Here's how the part is built. I have some questions about the finished solid (model axes, mm). Round coordinates to 2 decimals unless told otherwise and drop trailing zeros. Loops run counter-clockwise (first coordinate to the right, second up) from the corner with the lowest first, then second, coordinate; pieces in that order, holes last. Notation, with made-up numbers: M 74.25,6.5 L 120.25,6.5 A20 cw 120.25,38.5 Z; hole C 47,-23.5 d3. An arc over 180 degrees is marked long. Write item = value, one per line. Start each with the question number.
from build123d import *

# Parameters (mm, degrees)
F0_W     = 50
F0_H     = 80
F1_DEPTH = 10
F2_R     = 9
F3_DEPTH = 10.001
F4_R     = 5


with BuildPart() as f1:
    # F0 (on Front) → F1 (new body)
    with BuildSketch(Plane.XZ):
        with Locations((25, -40)):
            Rectangle(F0_W, F0_H)
    extrude(amount=F1_DEPTH)

    # F2 (on face) → F3 (cut, through all)
    with BuildSketch(Plane.XZ.offset(10)):
        with Locations((25, -40)):
            Circle(F2_R)
    extrude(amount=-F3_DEPTH, mode=Mode.SUBTRACT)

    # F4
    f4_edges = [f1.edges().sort_by_distance(p)[0] for p in [
        (50, -5, 0),
        (0, -5, 0),
        (50, -5, -80),
        (0, -5, -80),
    ]]
    fillet(f4_edges, radius=F4_R)


solid = f1.part
Item 1: Please list where these lines run through material, in increasing order: line 1 (Z direction, x = 25, y = -6.5); line 2 (Z direction, x = 32, y = -7.25); line 3 (X direction, y = -3.75, z = -41.5). Write a range as [from, to].
Item 2: I want a section at B-B, the plane y = -5.75. List the corners of the cut face in (x, z) for me.
Item 3: I want a section at A-A, the plane z = -40. List the corners of the cut face in (x, y) for me, then the cut area to 3 significant figures.
Item 4: We'd pull the mould along X, two halves only. Please class faces 1 (the cylindrical face through (29.84, -5.07, -32.41)), 2 (the flat face through (25, -5, 0)), 3 (the flat face through (50, -5, -40)): released by +X, released by -X, zero draft, split by the parting line, or undercut.
Item 5: I want a section at C-C, the plane x = 25. List the corners of the cut face in (y, z) for me.
Item 6: Will this pin go through, and if not, where does the flat tip stop? pin 1 Ø23.5 at (x, z) = (25, -40) entering from +Y.
Worked out:
q1.line_1 = [-80, -49], [-31, 0]
q1.line_2 = [-80, -45.66], [-34.34, 0]
q1.line_3 = [0, 16.13], [33.87, 50]
q2.outline = M 0,-75 A5 ccw 5,-80 L 45,-80 A5 ccw 50,-75 L 50,-5 A5 ccw 45,0 L 5,0 A5 ccw 0,-5 Z; hole C 25,-40 d18
q3.outline = M 0,-10 L 16,-10 L 16,0 L 0,0 Z; M 34,-10 L 50,-10 L 50,0 L 34,0 Z
q3.area = 320 mm2
q4.face_1 = undercut
q4.face_2 = zero draft
q4.face_3 = released by +X
q5.outline = M -10,-80 L 0,-80 L 0,-49 L -10,-49 Z; M -10,-31 L 0,-31 L 0,0 L -10,0 Z
q6.pin_1 = 0
